```python
from build123d import *

# Parameters (mm, degrees)
SKETCH1_W           = 40
SKETCH1_H           = 80
SKETCH1_W_2         = 37.6
SKETCH1_H_2         = 77.6
BOSS_EXTRUDE1_DEPTH = 1955
SKETCH2_R           = 11
CUT_EXTRUDE1_DEPTH  = 1955
SKETCH3_R           = 4.75
CUT_EXTRUDE2_DEPTH  = 1958.044966269
SKETCH4_R           = 3.5
CUT_EXTRUDE3_DEPTH  = 1958.044966269


with BuildPart() as part:
    # Sketch1 → Boss-Extrude1 (new body)
    with BuildSketch(Plane.XY):
        with Locations((20, 40)):
            Rectangle(SKETCH1_W, SKETCH1_H)
        with Locations((20, 40)):
            Rectangle(SKETCH1_W_2, SKETCH1_H_2, mode=Mode.SUBTRACT)
    extrude(amount=BOSS_EXTRUDE1_DEPTH)

    # Sketch2 → Cut-Extrude1 (cut)
    with BuildSketch(Plane(origin=(0, 80, 0), x_dir=(1, 0, 0), z_dir=(0, 1, 0))):
        with Locations(Location((20, -70, 0), (0, 0, 270))):
            Circle(SKETCH2_R)
        with BuildLine():
            Line((0, 0), (40, 0))
            ThreePointArc((40, 0), (20, -7.639320225), (0, 0))
        make_face()
        with BuildLine():
            Line((0, -1955), (40, -1955))
            ThreePointArc((40, -1955), (20, -1947.360679775), (0, -1955))
        make_face()
    extrude(amount=-CUT_EXTRUDE1_DEPTH, mode=Mode.SUBTRACT)

    # Sketch3 → Cut-Extrude2 (cut, through all)
    with BuildSketch(Plane(origin=(40, 0, 0), x_dir=(0, 0, -1), z_dir=(1, 0, 0))):
        with Locations((-17, 67.5)):
            Circle(SKETCH3_R)
        with Locations((-17, 12.5)):
            Circle(SKETCH3_R)
        with Locations((-1938, 67.5)):
            Circle(SKETCH3_R)
        with Locations((-1938, 12.5)):
            Circle(SKETCH3_R)
    extrude(amount=-CUT_EXTRUDE2_DEPTH, mode=Mode.SUBTRACT)

    # Sketch4 → Cut-Extrude3 (cut, through all)
    with BuildSketch(Plane(origin=(40, 0, 0), x_dir=(0, 0, -1), z_dir=(1, 0, 0))):
        with Locations((-1451.5, 60)):
            Circle(SKETCH4_R)
        with Locations((-1451.5, 20)):
            Circle(SKETCH4_R)
        with Locations((-503.5, 60)):
            Circle(SKETCH4_R)
        with Locations((-503.5, 20)):
            Circle(SKETCH4_R)
    extrude(amount=-CUT_EXTRUDE3_DEPTH, mode=Mode.SUBTRACT)


solid = part.part
```
CAD build for the part. Positions are in the model's coordinates, mm. A direction names the side the tool comes from. Give positions to 0.01 mm unless a question says otherwise; leave off trailing zeros. Write each loop counter-clockwise with the first axis right and the second up, starting at its lowest first coordinate (ties: lowest second). Pieces come first, ordered by that corner, then holes. Notation, with made-up numbers: M 30.5,14 L 81.5,14 A22 cw 81.5,24 Z; hole C 45,-17 d6. An arc over 180 degrees is marked long. Return JSON: item names as keys, results as strings. Group by question number.
(1) Mould opens along X. For faces 3 (the face through (0, 39, 964)), 4 (the face through (39.466, 40.187, 0.466)), 5 (the face through (40, 39, 964)) say: pulls with the +X half, pulls with the -X half, needs draft (parallel to the pull), parting line crosses it, or undercut.
(2) 3-axis set-ups, long thin cutter, end or side, ignore diameter. For faces 1 (the face through (20, 1.2, 964)), 2 (the face through (39.466, 40.187, 1954.534)): which of +Z, -Z, +X, -X, +Y, -Y reach the whole face in a straight line?
(3) Band-saw the part on A-A (z = 1409). Give the cut face in (x, y), and give its area (3 significant figures).
(4) Drill centre lines: L1, parallel to X at y = 60, z = 1171.5; L2, parallel to Y at x = 17.5, z = 834.5; L3, parallel to Y at x = 39.7, z = 17. Where is each one in solid material? Low to high. Write a range as [from, to].
(5) Flat gauge pins, fed straight in: pin 1 Ø5.5 at (y, z) = (20, 503.5) entering from -X; pin 2 Ø12 at (y, z) = (14, 412.5) entering from -X. Where does each tip first touch, or does it go through?
Entries:
{
 "1": {"face 3": "pulls with the -X half", "face 4": "undercut", "face 5": "pulls with the +X half"},
 "2": {"face 1": "+Z, -Z", "face 2": "+Z, +Y, -Y"},
 "3": {"outline": "M 0,0 L 40,0 L 40,80 L 0,80 Z; hole M 1.2,1.2 L 38.8,1.2 L 38.8,78.8 L 1.2,78.8 Z", "area": "282 mm^2"},
 "4": {"L1": "x = [0, 1.2], [38.8, 40]", "L2": "y = [0, 1.2], [78.8, 80]", "L3": "y = [0, 7.75], [17.25, 62.75], [72.25, 80]"},
 "5": {"pin 1": "passes through", "pin 2": "stops at x = 0"}
}
